For this review, use the dimensioned drawing (mm, ordinates from the lowest corner) and the shaded views. A direction names the side the tool comes from. Give positions to 0.01 mm unless a question says otherwise; leave off trailing zeros. Loops run counter-clockwise (first coordinate to the right, second up) from the corner with the lowest first, then second, coordinate; pieces in that order, holes last. Notation, with made-up numbers: M -32,-25 L -3,-25 A23 cw -3,-5 Z; hole C 27,-4.5 d1. An arc over 180 degrees is marked long. Return JSON: item names as keys, results as strings.
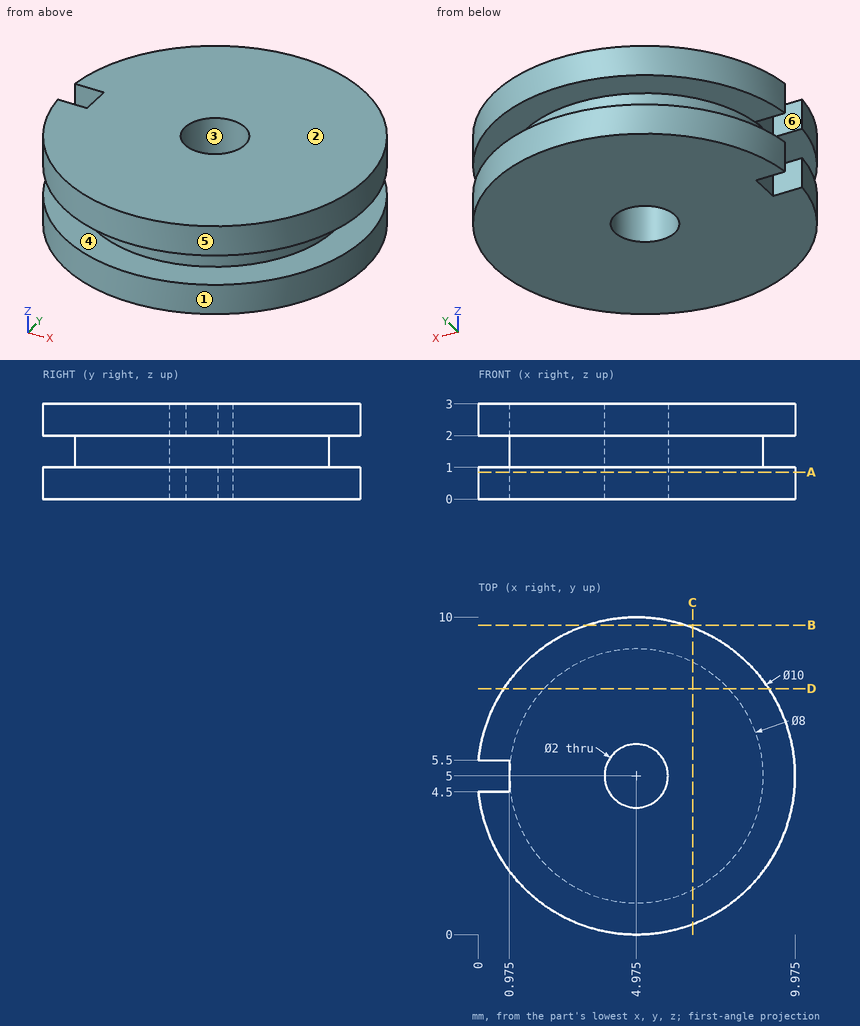
1) Consider section A-A on z = 0.85. Write out the cut boundary in (x, y) (3 decimals), then the cut area to 3 significant figures.
From the geometry:
{"outline": "M 0,4.5 A5 ccw long 0,5.5 L 0.975,5.5 L 0.975,4.5 Z; hole C 4.975,5 d2", "area": "74.4 mm²"}
2) Consider section D-D on y = 7.75. Write out the cut boundary in (x, z), then the cut area to 3 significant figures.
From the geometry:
{"outline": "M 0.8,0 L 9.15,0 L 9.15,1 L 7.88,1 L 7.88,2 L 9.15,2 L 9.15,3 L 0.8,3 L 0.8,2 L 2.07,2 L 2.07,1 L 0.8,1 Z", "area": "22.5 mm²"}
3) Tool access review of the marked faces 4, 5 and 6: name each direction out of +Z, -Z, +X, -X, +Y, -Y from which nothing blocks a thin tool from reaching the whole face with its end or side.
From the geometry:
{"face 4": "none", "face 5": "+Z, -Z", "face 6": "+Z, -Z, -X"}
4) Insertion check: pin 1 (0.5 mm diameter, centred on x = 0.5, z = 0.5, fed in from +Y); pin 2 (1.2 mm diameter, centred on x = 4.97, y = 5, fed in from +Z); pin 3 (1.1 mm diameter, centred on x = 0.5, z = 0.5, fed in from -Y); pin 4 (0.5 mm diameter, centred on y = 5, z = 0.5, fed in from -X) (3 decimals). Each pin has a flat end and moves straight along its axis. Give the tip position at first contact, or say it passes through.
From the geometry:
{"pin 1": "y = 7.67", "pin 2": "through", "pin 3": "y = 1.9", "pin 4": "x = 0.975"}
5) Consider section C-C on x = 6.75. Write out the cut boundary in (y, z).
From the geometry:
{"outline": "M 0.33,0 L 9.67,0 L 9.67,1 L 8.58,1 L 8.58,2 L 9.67,2 L 9.67,3 L 0.33,3 L 0.33,2 L 1.42,2 L 1.42,1 L 0.33,1 Z"}
6) Consider section B-B on y = 9.75. Write out the cut boundary in (x, z).
From the geometry:
{"outline": "M 3.41,0 L 6.54,0 L 6.54,1 L 3.41,1 Z; M 3.41,2 L 6.54,2 L 6.54,3 L 3.41,3 Z"}
7) Wall thickness on L1, parallel to Z at x = 6, y = 9.25; L2, parallel to X at y = 2, z = 2.15 (3 decimals); L3, parallel to X at y = 4.25, z = 2.7: over which ranges is each line inside the solid? List them lowest first. Write a range as from..to.
From the geometry:
{"L1": "0..1, 2..3", "L2": "0.975..8.975", "L3": "0.03..4.31, 5.64..9.92"}
8) The part is to be moulded in two halves that separate along Y. For the marked faces 1, 2 and 3, say which applies: released by +Y, released by -Y, zero draft, split by the parting line, or undercut.
From the geometry:
{"face 1": "split by the parting line", "face 2": "zero draft", "face 3": "undercut"}
